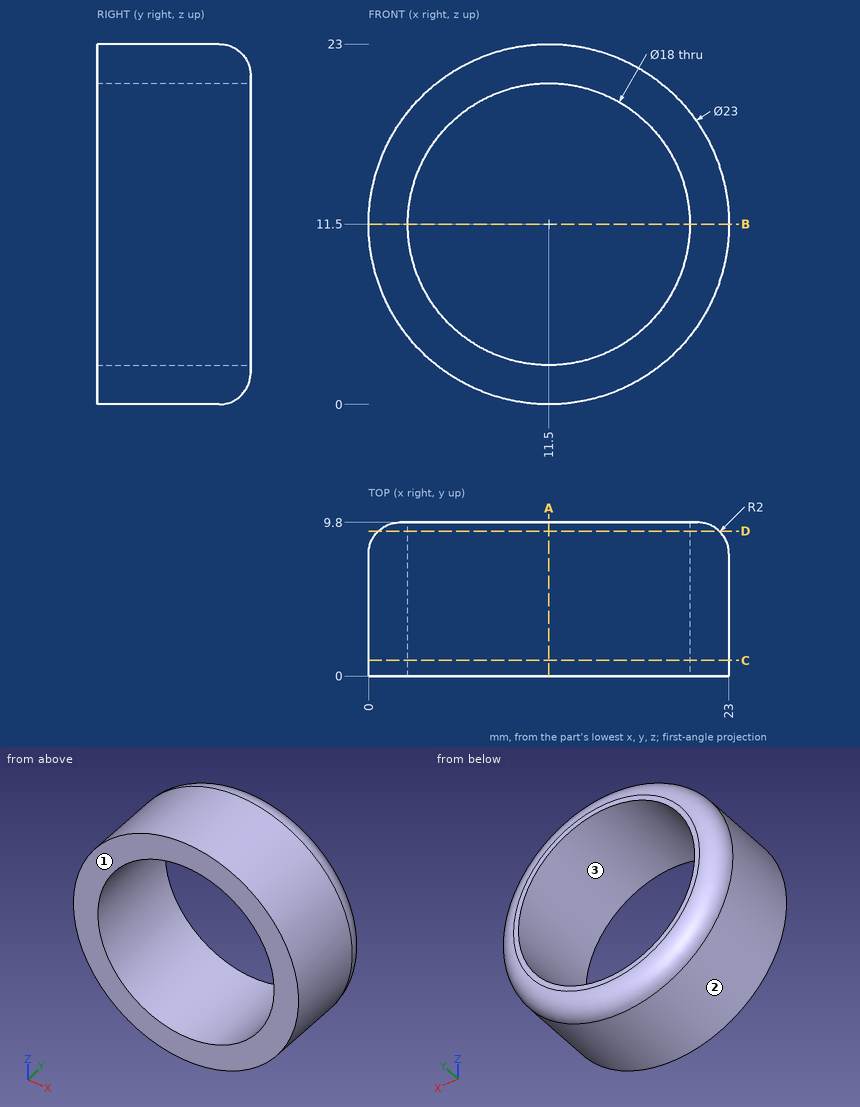
For this review, use the dimensioned drawing (mm, ordinates from the lowest corner) and the shaded views. Round coordinates to 2 decimals unless told otherwise and drop trailing zeros. Write each loop counter-clockwise with the first axis right and the second up, starting at its lowest first coordinate (ties: lowest second). Pieces come first, ordered by that corner, then holes. Notation, with made-up numbers: M 55,59.5 L 74,59.5 A13 ccw 74,84.5 Z; hole C 6.25,35 d9. An arc over 180 degrees is marked long. Use CSV: the item, a comma, the result in double quotes. Start each with the question number.
(1) We need section D-D, the plane y = 9.25. State the section outline as (x, z) points (1 decimal).
(2) Clearance check with flat-ended pins moving along their axes: P1, Ø8, axis at x = 6.5, z = 13.5, coming from the -Y side; P2, Ø8, axis at x = 10.5, z = 7.5, coming from the -Y side; P3, Ø5, axis at y = 2, z = 2.5, coming from the -X side; P4, Ø3, axis at y = 4.5, z = 15, coming from the -X side. State where each tip first meets the part, or that it passes through.
(3) We need section C-C, the plane y = 1. State the section outline as (x, z) points, then the cut area to 3 significant figures.
(4) The part is to be moulded in two halves that separate along Z. For the marked faces 1, 2 and 3, say which applies: +Z half, -Z half, draft (parallel to the pull), parting line (faces both ways), or undercut.
(5) For line 1 along Z through (x, y) = (11.5, 5.25); line 2 along Z through (x, y) = (18, 1); line 3 along X through (y, z) = (1, 3.5), list the stretches that pass through material, from the lowest coordinate up.
(6) We need section A-A, the plane x = 11.5. State the section outline as (y, z) points, then the cut area to 3 significant figures.
(7) We need section B-B, the plane z = 11.5. State the section outline as (x, y) points.
Findings:
1,outline,"C 11.5,11.5 d21.8; hole C 11.5,11.5 d18"
2,P1,"y = 0"
2,P2,"through"
2,P3,"x = 2.01"
2,P4,"x = 0.18"
3,outline,"C 11.5,11.5 d23; hole C 11.5,11.5 d18"
3,area,"161 mm^2"
4,face 1,"draft"
4,face 2,"parting line"
4,face 3,"undercut"
5,line 1,"0 to 2.5, 20.5 to 23"
5,line 2,"2.01 to 5.28, 17.72 to 20.99"
5,line 3,"3.24 to 7.38, 15.62 to 19.76"
6,outline,"M 0,0 L 7.8,0 A2 ccw 9.8,2 L 9.8,2.5 L 0,2.5 Z; M 0,20.5 L 9.8,20.5 L 9.8,21 A2 ccw 7.8,23 L 0,23 Z"
6,area,"47.3 mm^2"
7,outline,"M 0,0 L 2.5,0 L 2.5,9.8 L 2,9.8 A2 ccw 0,7.8 Z; M 20.5,0 L 23,0 L 23,7.8 A2 ccw 21,9.8 L 20.5,9.8 Z"
